Part print with two shaded views. Sizes in mm from the minimum x, y, z corner. Round coordinates to 2 decimals unless told otherwise and drop trailing zeros. Order: outer loops, then holes, each group sorted by start corner. A loop starts at its lowest first (then second) coordinate and runs counter-clockwise, first axis right, second up. Notation, with made-up numbers: M 68.5,24 L 126.5,24 A20 cw 126.5,42 Z; hole C 57,-8 d1. An arc over 180 degrees is marked long. Put each result on its own line as item: value.
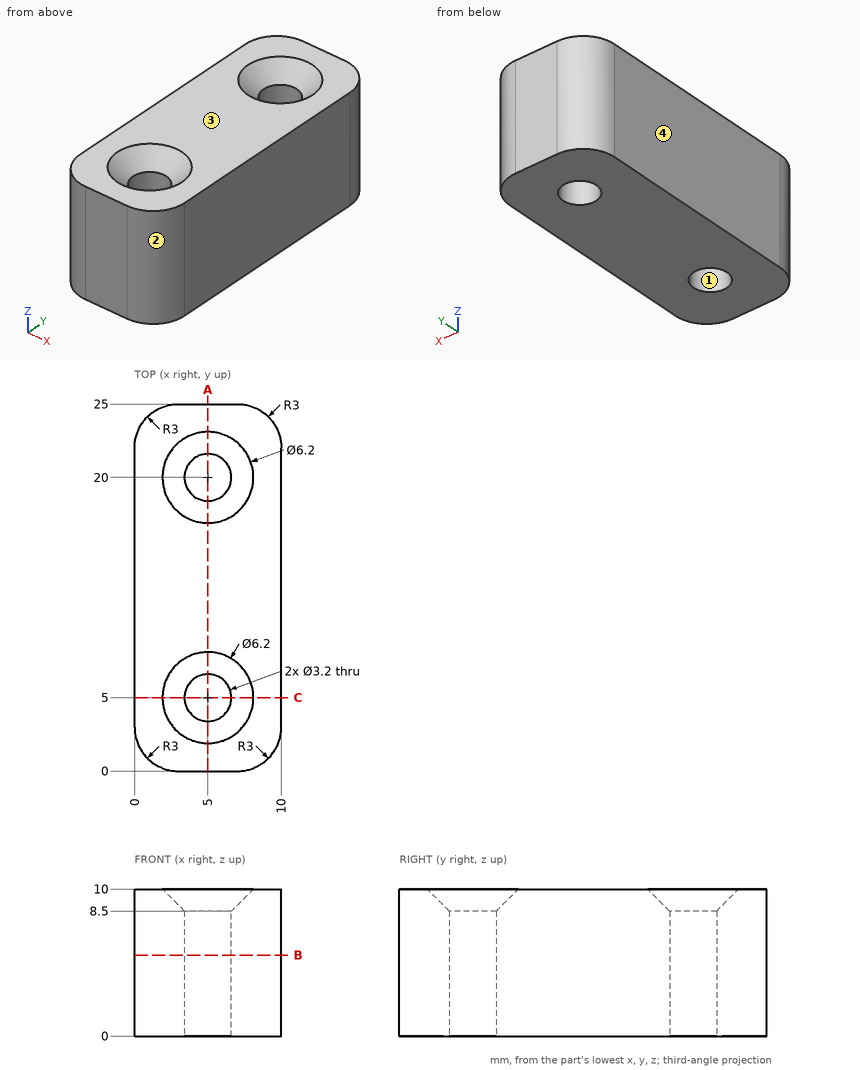
Item 1: Mould opens along X. For the marked faces 1, 2, 3 and 4 say: pulls with the +X half, pulls with the -X half, needs draft (parallel to the pull), parting line crosses it, or undercut.
Answers below:
face 1: undercut
face 2: pulls with the +X half
face 3: needs draft
face 4: pulls with the -X half
Item 2: Band-saw the part on C-C on y = 5. Give the cut face in (x, z), and give its area (4 significant figures).
Answers below:
outline: M 0,0 L 3.4,0 L 3.4,8.5 L 1.9,10 L 0,10 Z; M 6.6,0 L 10,0 L 10,10 L 8.1,10 L 6.6,8.5 Z
area: 65.75 mm²
Item 3: Pin check, flat tips, straight feed: P1, Ø4, axis at x = 5, y = 20, coming from the +Z side; P2, Ø5, axis at y = 17, z = 5, coming from the -X side. Stop position of each tip, or through.
Answers below:
P1: z = 8.9
P2: x = 0
Item 4: Band-saw the part on A-A on x = 5. Give the cut face in (y, z), and give its area (4 significant figures).
Answers below:
outline: M 0,0 L 3.4,0 L 3.4,8.5 L 1.9,10 L 0,10 Z; M 6.6,0 L 18.4,0 L 18.4,8.5 L 16.9,10 L 8.1,10 L 6.6,8.5 Z; M 21.6,0 L 25,0 L 25,10 L 23.1,10 L 21.6,8.5 Z
area: 181.5 mm²
Item 5: Probe line 1 along Y through (x, z) = (5, 4.5); line 2 along Y through (x, z) = (6.25, 4.5); line 3 along X through (y, z) = (4.5, 9.5). List the from-to ranges inside material, lowest first. Write a range as [from, to].
Answers below:
line 1: [0, 3.4], [6.6, 18.4], [21.6, 25]
line 2: [0, 4], [6, 19], [21, 25]
line 3: [0, 2.45], [7.55, 10]
Item 6: Band-saw the part on B-B on z = 5.5. Give the cut face in (x, y).
Answers below:
outline: M 0,3 A3 ccw 3,0 L 7,0 A3 ccw 10,3 L 10,22 A3 ccw 7,25 L 3,25 A3 ccw 0,22 Z; hole C 5,5 d3.2; hole C 5,20 d3.2
